Work out the finished part from the listing and answer in its coordinate system (mm). Face numbers are marked on the shaded views. A direction names the side the tool comes from. Coordinates: 2 decimals unless noted, no trailing zeros. Order: outer loops, then holes, each group sorted by start corner. A loop starts at its lowest first (then second) coordinate and runs counter-clockwise, first axis right, second up. Notation, with made-up numbers: M 8,81 L 31,81 A13 cw 31,99 Z; hole C 28.25,29 d6. An arc over 180 degrees is marked long. Answer in a Markdown table with one row per item. Add a question column.
Item 1: The part is cut by section B-B (y = 38). Write down the section's boundary in (x, z), then the cut area to 3 significant figures.
Item 2: Consider line 1 (X direction, y = 13, z = 70); line 2 (X direction, y = 6, z = 72); line 3 (X direction, y = 1.25, z = 44). Determine where each line is inside the solid, lowest interval first. Write a range as from..to.
Item 3: Flat-ended cylindrical pins translate along their axes: pin 1 Ø1.5 at (x, z) = (1.5, 31.5) entering from +Y; pin 2 Ø4 at (x, z) = (69, 72.5) entering from +Y; pin 3 Ø21 at (y, z) = (35, 39) entering from +X. Find the tip coordinate at first contact, or state that the pin passes through.
Item 4: The part is cut by section C-C (x = 48.36). Write down the section's boundary in (y, z), then the cut area to 4 significant figures.
Item 5: The part is cut by section A-A (z = 44). Write down the section's boundary in (x, y), then the cut area to 3 significant figures.
Item 6: Which of the six approach directions +Z, -Z, +X, -X, +Y, -Y give full straight-line access (tool end or side, diameter ignored) to the marked faces 1, 2, 3, 4 and 5?
Item 7: The part is cut by section D-D (y = 15.5). Write down the section's boundary in (x, z), then the cut area to 3 significant figures.
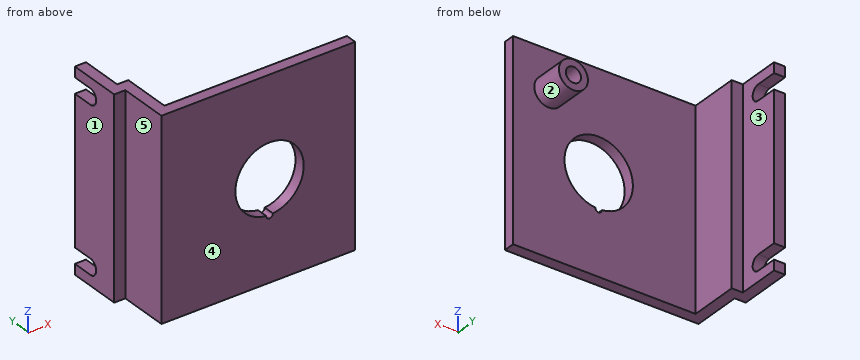
from build123d import *

# Parameters (mm, degrees)
P_IDAT_VYSUNUT_M1_DEPTH  = 88
ODEBRAT_VYSUNUT_M1_REACH = 93.66
ODEBRAT_VYSUNUT_M2_REACH = 48
SKICA4_R                 = 6.5
P_IDAT_VYSUNUT_M2_DEPTH  = 15
M8_Z_VIT1_D              = 6.8
M8_Z_VIT1_DEPTH          = 14
M8_Z_VIT1_TIP            = 2.042926105


with BuildPart() as part:
    # Skica1 → Přidat vysunutím1 (new body)
    with BuildSketch(Plane.XY):
        Polygon((0, 0), (0, 22), (-5, 22), (-5, 46), (0, 46), (0, 27), (5, 27), (5, 5), (86.66, 5), (86.66, 0), align=None)
    extrude(amount=P_IDAT_VYSUNUT_M1_DEPTH)

    # Skica2 → Odebrat vysunutím1 (cut, up to next)
    with BuildSketch(Plane.ZY.offset(5), mode=Mode.PRIVATE) as odebrat_vysunut_m1_sk1:
        with BuildLine():
            Line((4.6, 46), (4.6, 36.45))
            ThreePointArc((4.6, 36.45), (8.05, 33), (11.5, 36.45))
            Line((11.5, 36.45), (11.5, 46))
            Line((11.5, 46), (4.6, 46))
        make_face()
    odebrat_vysunut_m1_tool1 = extrude(odebrat_vysunut_m1_sk1.sketch, amount=-ODEBRAT_VYSUNUT_M1_REACH, mode=Mode.PRIVATE) & part.part
    add(odebrat_vysunut_m1_tool1.solids().sort_by_distance((-5, 39.846006, 8.05))[0], mode=Mode.SUBTRACT)
    # Skica2 → Odebrat vysunutím1 (cut, up to next)
    with BuildSketch(Plane.ZY.offset(5), mode=Mode.PRIVATE) as odebrat_vysunut_m1_sk2:
        with BuildLine():
            Line((83.4, 46), (76.5, 46))
            Line((76.5, 46), (76.5, 36.45))
            ThreePointArc((76.5, 36.45), (79.95, 33), (83.4, 36.45))
            Line((83.4, 36.45), (83.4, 46))
        make_face()
    odebrat_vysunut_m1_tool2 = extrude(odebrat_vysunut_m1_sk2.sketch, amount=-ODEBRAT_VYSUNUT_M1_REACH, mode=Mode.PRIVATE) & part.part
    add(odebrat_vysunut_m1_tool2.solids().sort_by_distance((-5, 39.846006, 79.95))[0], mode=Mode.SUBTRACT)

    # Skica3 → Odebrat vysunutím2 (cut, up to next)
    with BuildSketch(Plane.XZ, mode=Mode.PRIVATE) as odebrat_vysunut_m2_sk1:
        with BuildLine():
            ThreePointArc((49.858196725, 28.773529412), (48.36, 59.3), (46.861803275, 28.773529412))
            ThreePointArc((46.861803275, 28.773529412), (48.36, 27.2), (49.858196725, 28.773529412))
        make_face()
    odebrat_vysunut_m2_tool1 = extrude(odebrat_vysunut_m2_sk1.sketch, amount=-ODEBRAT_VYSUNUT_M2_REACH, mode=Mode.PRIVATE) & part.part
    add(odebrat_vysunut_m2_tool1.solids().sort_by_distance((48.36, 0, 43.922265))[0], mode=Mode.SUBTRACT)

    # Skica4 → Přidat vysunutím2 (add)
    with BuildSketch(Plane(origin=(0, 5, 0), x_dir=(1, 0, 0), z_dir=(0, 1, 0))):
        with Locations((70.66, -70)):
            Circle(SKICA4_R)
    extrude(amount=P_IDAT_VYSUNUT_M2_DEPTH)

    # M8 závit1
    with Locations(Plane(origin=(0, 20, 0), x_dir=(1, 0, 0), z_dir=(0, 1, 0))):
        with Locations((70.66, -70)):
            Hole(M8_Z_VIT1_D / 2, depth=M8_Z_VIT1_DEPTH)
            with Locations((0, 0, -(M8_Z_VIT1_DEPTH + M8_Z_VIT1_TIP / 2))):  # 118° drill point
                Cone(0, M8_Z_VIT1_D / 2, M8_Z_VIT1_TIP, mode=Mode.SUBTRACT)


solid = part.part
Reply:
| question | item | result |
|---|---|---|
| 1 | outline | M -5,0 L 0,0 L 0,4.6 L -5,4.6 Z; M -5,11.5 L 0,11.5 L 0,76.5 L -5,76.5 Z; M -5,83.4 L 0,83.4 L 0,88 L -5,88 Z |
| 1 | area | 371 mm2 |
| 2 | line 1 | x = 0..5, 64.16..67.26, 74.06..77.16 |
| 2 | line 2 | x = 0..5, 64.48..67.91, 73.41..76.84 |
| 2 | line 3 | x = 0..33.06, 63.66..86.66 |
| 3 | pin 1 | stops at y = 27 |
| 3 | pin 2 | stops at y = 20 |
| 3 | pin 3 | stops at x = 5 |
| 4 | outline | M 0,0 L 5,0 L 5,27.2 L 0,27.2 Z; M 0,59.3 L 5,59.3 L 5,88 L 0,88 Z |
| 4 | area | 279.5 mm2 |
| 5 | outline | M -5,22 L 0,22 L 0,0 L 33.06,0 L 33.06,5 L 5,5 L 5,27 L 0,27 L 0,46 L -5,46 Z; M 63.66,0 L 86.66,0 L 86.66,5 L 63.66,5 Z |
| 5 | area | 510 mm2 |
| 6 | face 1 | +Z, -Z, -X, +Y, -Y |
| 6 | face 2 | +Y |
| 6 | face 3 | +Z, -Z, +X, +Y |
| 6 | face 4 | +Z, -Z, +X, -X, -Y |
| 6 | face 5 | +Z, -Z, -X, -Y |
| 7 | outline | M 0,0 L 5,0 L 5,88 L 0,88 Z; C 70.66,70 d13; hole C 70.66,70 d6.8 |
| 7 | area | 536 mm2 |
